For this review, take the finished solid that the model builds, in its own axes (mm). Face numbers are marked on the shaded views. A direction names the side the tool comes from. Give positions to 0.01 mm unless a question says otherwise; leave off trailing zeros. Order: outer loops, then holes, each group sorted by start corner. A loop starts at its lowest first (then second) coordinate and runs counter-clockwise, first axis right, second up. Notation, with made-up numbers: (12, -38.5) - (34, -38.5) arc R29 ccw to (34, -4.5) - close; hole circle Ø6 at (-30.5, -29). An arc over 180 degrees is marked (long way). Use a Markdown table: item, result. Add a question column.
1) We need section B-B on z = -0.8. Write out the cut boundary in (x, y), then the cut area to 3 significant figures.
2) We need section C-C on x = 0.75. Write out the cut boundary in (y, z).
3) We need section A-A on x = -4.5. Write out the cut boundary in (y, z).
4) Wall thickness on L1, parallel to Z at x = -2, y = 0; L2, parallel to X at y = 0.5, z = 0.25; L3, parallel to Y at x = 2, z = -0.3: over which ranges is each line inside the solid? List them lowest first.
5) Mouldability with a two-part tool opening along Y and no side actions: class the marked faces 1, 2, 3 and 4 as released by +Y, released by -Y, zero draft, split by the parting line, or undercut.
6) Machinability: for the marked faces 5 and 6, which of the approach directions +Z, -Z, +X, -X, +Y, -Y give a long, thin tool a straight path to every point of the face, cutting with its end or side? Answer none if there is none.
7) We need section D-D on y = 4.75. Write out the cut boundary in (x, z), then the cut area to 3 significant figures.
```python
from build123d import *

# Parameters (mm, degrees)
BOSS_EXTRUDE1_DEPTH = 2
BOSS_EXTRUDE2_DEPTH = 0.7


with BuildPart() as part:
    # Sketch1 → Boss-Extrude1 (new body)
    with BuildSketch(Plane.XY):
        Polygon((0, -6.142777017), (2.175697935, -3.768419365), (5.319800946, -3.071388508), (4.351395869, 0), (5.319800946, 3.071388508), (2.175697935, 3.768419365), (0, 6.142777017), (-2.175697935, 3.768419365), (-5.319800946, 3.071388508), (-4.351395869, 0), (-5.319800946, -3.071388508), (-2.175697935, -3.768419365), align=None)
    extrude(amount=-BOSS_EXTRUDE1_DEPTH)

    # Sketch1_4 → Boss-Extrude2 (add)
    with BuildSketch(Plane.XY):
        with BuildLine():
            ThreePointArc((1.15, 0), (0.813172798, 0.813172798), (0, 1.15))
            Line((0, 1.15), (0, -1.15))
            ThreePointArc((0, -1.15), (0.813172798, -0.813172798), (1.15, 0))
        make_face()
        with BuildLine():
            Line((0, -1.15), (0, 1.15))
            ThreePointArc((0, 1.15), (-1.15, 0), (0, -1.15))
        make_face()
    extrude(amount=BOSS_EXTRUDE2_DEPTH)


solid = part.part
```
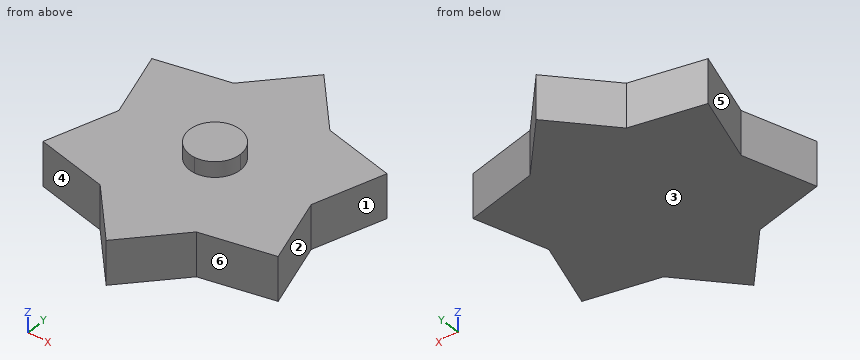
Checked values:
| question | item | result |
|---|---|---|
| 1 | outline | (-5.32, -3.07) - (-2.18, -3.77) - (0, -6.14) - (2.18, -3.77) - (5.32, -3.07) - (4.35, 0) - (5.32, 3.07) - (2.18, 3.77) - (0, 6.14) - (-2.18, 3.77) - (-5.32, 3.07) - (-4.35, 0) - close |
| 1 | area | 80.2 mm² |
| 2 | outline | (-5.32, -2) - (5.32, -2) - (5.32, 0) - (0.87, 0) - (0.87, 0.7) - (-0.87, 0.7) - (-0.87, 0) - (-5.32, 0) - close |
| 3 | outline | (-3.25, -2) - (-0.47, -2) - (-0.47, 0) - (-3.25, 0) - close; (0.47, -2) - (3.25, -2) - (3.25, 0) - (0.47, 0) - close |
| 4 | L1 | -2 to 0 |
| 4 | L2 | -1.04 to 1.04 |
| 4 | L3 | -3.96 to 3.96 |
| 5 | face 1 | undercut |
| 5 | face 2 | undercut |
| 5 | face 3 | zero draft |
| 5 | face 4 | released by -Y |
| 6 | face 5 | +Z, -Z, -X |
| 6 | face 6 | +Z, -Z, +X, -Y |
| 7 | outline | (-1.28, -2) - (1.28, -2) - (1.28, 0) - (-1.28, 0) - close |
| 7 | area | 5.10 mm² |
